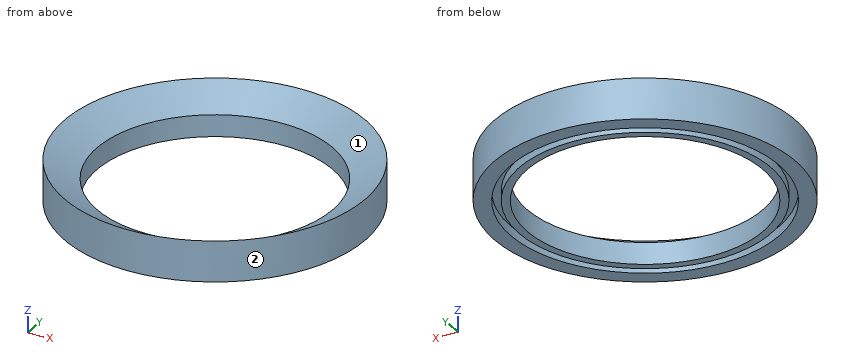
Autodesk Inventor part; units mm, degrees
ref_plane "YZ Plane" through (0, 0, 0) normal (1, 0, 0) x (0, 1, 0)
ref_plane "XZ Plane" through (0, 0, 0) normal (0, 1, 0) x (-1, 0, 0)
ref_plane "XY Plane" through (0, 0, 0) normal (0, 0, 1) x (1, 0, 0)
sketch "Sketch3" plane through (0, 0, 0) normal (0, 0, 1) x (1, 0, 0)
  circle A0 centre (0, 0) radius 55.5
  dimension "d5" = 111
sketch "Sketch4" plane through (0, 0, 0) normal (1, 0, 0) x (0, 1, 0)
  line L0 (55.5, 0) -> (-55.5, 0) construction
  line L1 (-55.5, 0) -> (-55.5, 15)
  line L2 (-55.5, 0) -> (-40.5, 0) construction
  line L3 (-55.5, 0) -> (-49.5, 0) construction
  line L4 (-49.5, 0) -> (-49.5, 3.5)
  line L5 (-49.5, 3.5) -> (-46.42, 3.5)
  line L6 (-49.5, 3.5) -> (-46.42, 3.5) construction
  line L7 (-46.42, 3.5) -> (-46.42, 0)
  line L8 (-46.42, 3.5) -> (-42.92, 3.5) construction
  line L9 (-46.42, 0) -> (-43.5, 0)
  line L10 (-43.5, 0) -> (-43.5, 8)
  line L11 (-43.5, 8) -> (-55.5, 15)
  line L12 (-55.5, 0) -> (-49.5, 0)
  line L13 (-49.5, 0) -> (-49.5, 3.5)
  line L14 (-43.5, 0) -> (-43.5, 8)
  line L15 (-43.5, 8) -> (-55.5, 15)
  line L16 (-55.5, 0) -> (-49.5, 0)
  line L17 (-49.5, 0) -> (-49.5, 3.5)
  line L18 (-46.42, 3.5) -> (-49.5, 3.5)
  line L19 (-46.42, 3.5) -> (-46.42, 0)
  line L20 (-46.42, 0) -> (-43.5, 0)
  point P0 (0, 0)
  dimension "d6" = 15
  dimension "d7" = 90
  dimension "d9" = 3.5
  dimension "d10" = 90
  dimension "d11" = 3.08
  dimension "d12" = 0
  dimension "d13" = 90
  dimension "d15" = 8
  dimension "d18" = 12
  dimension "d19" = 6
sweep "Sweep1" add profiles "Sketch4" path "Sketch3"
properties part number "Shaft"
Work out the finished part from the listing and answer in its coordinate system (mm). Face numbers are marked on the shaded views. Coordinates: 2 decimals unless noted, no trailing zeros. Loops run counter-clockwise (first coordinate to the right, second up) from the corner with the lowest first, then second, coordinate; pieces in that order, holes last. Notation, with made-up numbers: (-18.5, 5.5) -> (13.5, 5.5) arc R23 cw to (13.5, 37.5) -> close; hole circle Ø9 at (13, -33). An arc over 180 degrees is marked (long way). Write each question's results on one line, items separated by ' | '. Start each with the question number.
1) Consider line 1 along Y through (x, z) = (0, 0.8); line 2 along Y through (x, z) = (0, 3.75); line 3 along Y through (x, z) = (13.5, 1). Determine where each line is inside the solid, lowest interval first.
2) The mould has two halves that part along Y. Classify the marked faces 1 and 2: pulls with the +Y half, pulls with the -Y half, needs draft (parallel to the pull), parting line crosses it, or undercut.
3) Flat-ended cylindrical pins translate along their axes: P1, Ø6, axis at y = -24, z = 6, coming from the +X side; P2, Ø3, axis at x = -30.5, z = 2.5, coming from the -Y side; P3, Ø1, axis at x = -15.5, z = 6, coming from the -Y side. Find the tip coordinate at first contact, or state that the pin passes through.
4) Find section A-A on z = 5.25. Determine the outline of the cut face in (x, y), then the cut area to 3 significant figures.
Response values:
1) line 1: y = -55.5 to -49.5, -46.42 to -43.5, 43.5 to 46.42, 49.5 to 55.5 | line 2: y = -55.5 to -43.5, 43.5 to 55.5 | line 3: y = -53.83 to -47.62, -44.41 to -41.35, 41.35 to 44.41, 47.62 to 53.83
2) face 1: undercut | face 2: parting line crosses it
3) P1: stops at x = 51.37 | P2: stops at y = -47.32 | P3: stops at y = -53.43
4) outline: circle Ø111 at (0, 0); hole circle Ø87 at (0, 0) | area: 3,730 mm^2
